Input: part model. Units: mm. Frame: model coordinates. A direction names the side the tool comes from. Round coordinates to 2 decimals unless told otherwise and drop trailing zeros. Loops run counter-clockwise (first coordinate to the right, second up) from the corner with the lowest first, then second, coordinate; pieces in that order, holes last.
(1) Cut plane A-A, the plane y = 0. Output: boundary loops of the cut face in (x, z), and give its area (3 significant figures).
(2) Access query for faces 1 (the face through (-11.5, 0, -18)), 2 (the face through (-2.5, 34, -16)), 3 (the face through (-10, -13, 0)). Directions: +Z, -Z, +X, -X, +Y, -Y. A direction counts if a zero-diameter tool reaches every point of the face in a straight line with its end or side. Return the directions, or none.
(3) First-contact query: pin 1 Ø0.9 at (x, y) = (0.5, 21) entering from +Z; pin 2 Ø5 at (x, z) = (2, 6) entering from +Y; pin 3 Ø19.5 at (y, z) = (25, -17.5) entering from -X. Flat tips, straight axial feed; report the tip coordinate or a pass-through.
(4) Line query: line 1 (X direction, y = 24, z = -26); line 2 (Y direction, x = -3.5, z = -26); line 3 (Z direction, x = -17, y = -6). Output: solid intervals per line, ascending.
(5) Cut plane C-C, the plane x = 0. Output: boundary loops of the cut face in (y, z), and give its area (3 significant figures).
(6) Draft query along Z for faces 4 (the face through (-14.985, 0.66, 4.944)), 5 (the face through (-0.53, 33.34, -15.79)), 6 (the face through (0.021, 38.342, -16.356)), 7 (the face through (0, 12, -30)). Return one class per face: released by +Z, released by -Z, zero draft, split by the parting line, or undercut.
(7) Cut plane B-B, the plane z = -16. Give the number of separate pieces and of enclosed holes in the cut face, and give its area (3 significant figures).
from build123d import *

# Parameters (mm, degrees)
F0_R          = 15
F1_DEPTH      = 10
F2_R          = 20
F3_DEPTH      = 30
F5_DEPTH      = 2.5
F5_DEPTH_BACK = 2.5
F7_DEPTH      = 25
F8_W          = 23
F8_H          = 23
F9_DEPTH      = 25
F10_R         = 1


with BuildPart() as f1:
    # F0 (on Top) → F1 (new body)
    with BuildSketch(Plane.XY):
        Circle(F0_R)
    extrude(amount=F1_DEPTH)

    # F2 (on Top) → F3 (join)
    with BuildSketch(Plane.XY):
        Circle(F2_R)
    extrude(amount=-F3_DEPTH)

    # F4 (on Right) → F5 (join, two sides)
    with BuildSketch(Plane.YZ) as f5_sk:
        with BuildLine():
            ThreePointArc((24.3955058538, -30), (34.2598373067, -25.9140601285), (38.3457771782, -16.0497286756))
            ThreePointArc((38.3457771782, -16.0497286756), (34.2598373067, -6.1853972226), (24.3955058538, -2.0994573511))
            Line((24.3955058538, -2.0994573511), (17.0112717897, -7.5845918618))
            Line((17.0112717897, -7.5845918618), (15.4388935224, -5.3544416027))
            ThreePointArc((15.4388935224, -5.3544416027), (10.5016803992, -17.3033969985), (17.4980895184, -28.1755572213))
            Line((17.4980895184, -28.1755572213), (18.3211155236, -26.8716588616))
            Line((18.3211155236, -26.8716588616), (24.3955058538, -30))
        make_face()
        with BuildLine():
            Line((17.0112717897, -7.5845918618), (24.3955058538, -2.0994573511))
            ThreePointArc((24.3955058538, -2.0994573511), (19.6306389371, -2.9384315127), (15.4388935224, -5.3544416027))
            Line((15.4388935224, -5.3544416027), (17.0112717897, -7.5845918618))
        make_face()
        with BuildLine():
            ThreePointArc((15.4388935224, -5.3544416027), (19.6306389371, -2.9384315127), (24.3955058538, -2.0994573511))
            Line((24.3955058538, -2.0994573511), (13.1439510733, -2.0994573511))
            Line((13.1439510733, -2.0994573511), (15.4388935224, -5.3544416027))
        make_face()
        with BuildLine():
            Line((16.3464937359, -30), (24.3955058538, -30))
            ThreePointArc((24.3955058538, -30), (20.8281909127, -29.5361786954), (17.4980895184, -28.1755572213))
            Line((17.4980895184, -28.1755572213), (16.3464937359, -30))
        make_face()
        with BuildLine():
            ThreePointArc((17.4980895184, -28.1755572213), (20.8281909127, -29.5361786954), (24.3955058538, -30))
            Line((24.3955058538, -30), (18.3211155236, -26.8716588616))
            Line((18.3211155236, -26.8716588616), (17.4980895184, -28.1755572213))
        make_face()
    extrude(amount=F5_DEPTH)
    extrude(f5_sk.sketch, amount=-F5_DEPTH_BACK)

    # F6 (on face) → F7 (cut)
    with BuildSketch(Plane(origin=(-2.5, 0, 0), x_dir=(0, -1, 0), z_dir=(-1, 0, 0))):
        with BuildLine():
            Line((-19.843134833, -23.4803773318), (-19.843134833, -8.6190800193))
            ThreePointArc((-19.843134833, -8.6190800193), (-33.3457771782, -16.0497286756), (-19.843134833, -23.4803773318))
        make_face()
    extrude(amount=-F7_DEPTH, mode=Mode.SUBTRACT)

    # F8 (on face) → F9 (cut)
    with BuildSketch(Plane(origin=(0, 0, -30), x_dir=(1, 0, 0), z_dir=(0, 0, -1))):
        Rectangle(F8_W, F8_H)
    extrude(amount=-F9_DEPTH, mode=Mode.SUBTRACT)

    # F10
    f10_edges = [f1.edges().sort_by_distance(p)[0] for p in [
        (-15, 0, 10),
        (-20, 0, 0),
        (2.5, 22.11932, -2.099457),
        (-2.5, 38.345777, -16.049729),
        (2.5, 33.345777, -16.049729),
        (-15, 0, 0),
    ]]
    fillet(f10_edges, radius=F10_R)


solid = f1.part
Reported:
1. outline: (-20, -30) - (-11.5, -30) - (-11.5, -5) - (11.5, -5) - (11.5, -30) - (20, -30) - (20, -1) arc R1 ccw to (19, 0) - (16, 0) arc R1 cw to (15, 1) - (15, 9) arc R1 ccw to (14, 10) - (-14, 10) arc R1 ccw to (-15, 9) - (-15, 1) arc R1 cw to (-16, 0) - (-19, 0) arc R1 ccw to (-20, -1) - close
1. area: 925 mm2
2. face 1: -Z
2. face 2: +Z, -Z, -X, +Y
2. face 3: +Z
3. pin 1: stops at z = -2.1
3. pin 2: stops at y = 15
3. pin 3: stops at x = -12.94
4. line 1: x = -2.5 to 2.5
4. line 2: y = -19.69 to -11.5, 11.5 to 19.69
4. line 3: z = -30 to 0
5. outline: (-20, -30) - (-11.5, -30) - (-11.5, -5) - (11.5, -5) - (11.5, -30) - (24.4, -30) arc R13.95 ccw to (24.4, -2.1) - (20, -2.1) - (20, -1) arc R1 ccw to (19, 0) - (16, 0) arc R1 cw to (15, 1) - (15, 9) arc R1 ccw to (14, 10) - (-14, 10) arc R1 ccw to (-15, 9) - (-15, 1) arc R1 cw to (-16, 0) - (-19, 0) arc R1 ccw to (-20, -1) - close; hole (19.84, -23.48) arc R8.8 ccw (long way) to (19.84, -8.62) - close
5. area: 1,150 mm2
6. face 4: zero draft
6. face 5: undercut
6. face 6: split by the parting line
6. face 7: released by -Z
7. separate pieces: 2
7. enclosed holes: 1
7. area: 751 mm2
